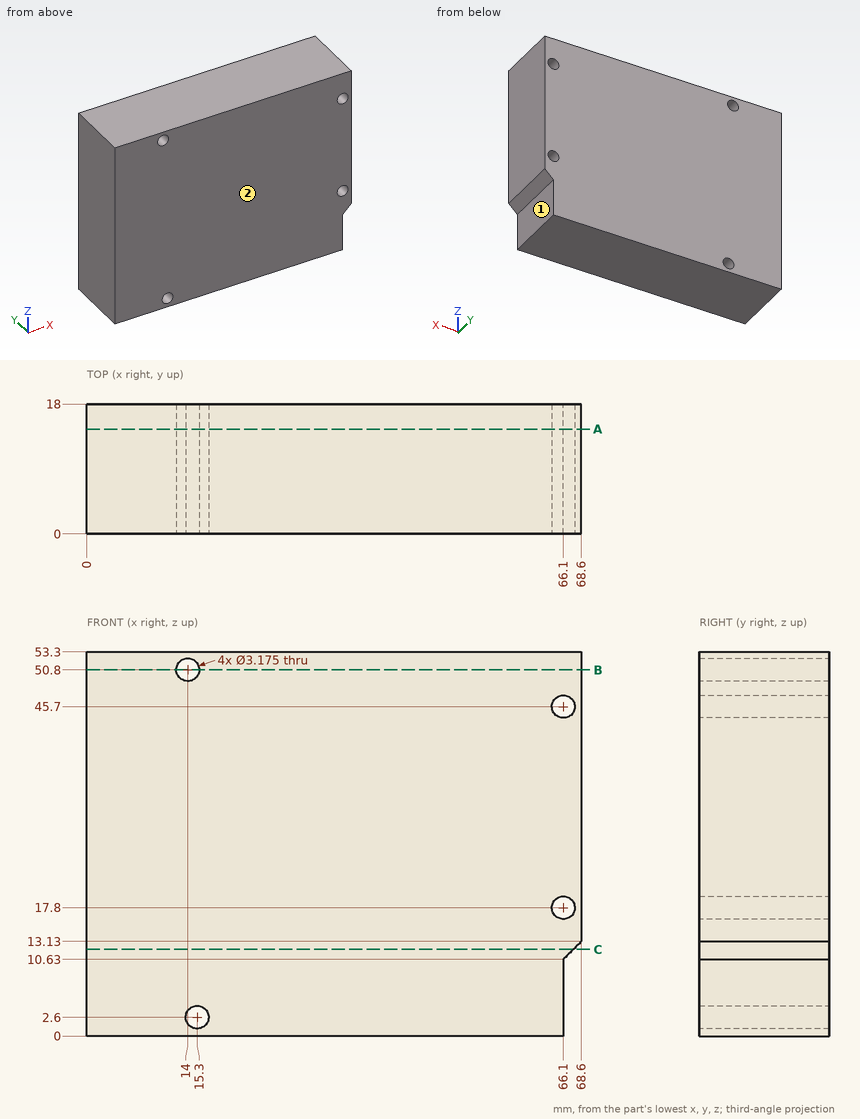
Geometry: see drawing. Coordinates: mm, zero at the bounding-box minimum. A direction names the side the tool comes from. Coordinates: 2 decimals unless noted, no trailing zeros. Write each loop counter-clockwise with the first axis right and the second up, starting at its lowest first coordinate (ties: lowest second). Pieces come first, ordered by that corner, then holes.
1) Set-up query: the marked faces 1 and 2. Return all of +Z, -Z, +X, -X, +Y, -Y with unobstructed straight access to the full face (end or side cutting, diameter ignored); none if empty.
2) Material intervals for line 1 along X through (y, z) = (6.25, 50.8); line 2 along X through (y, z) = (5.75, 2.6); line 3 along Z through (x, y) = (65, 15) (1 decimal), sorted ascending.
3) Section B-B on z = 50.8. Output: boundary loops of the cut face in (x, y).
4) Section C-C on z = 12. Output: boundary loops of the cut face in (x, y).
5) Section A-A on y = 14.5. Output: boundary loops of the cut face in (x, z) (1 decimal).
6) Pin query (flat end, axial travel): pin 1 Ø2.5 at (x, z) = (15.3, 2.6) entering from -Y. Return the tip coordinate at first contact, or that it passes through.
Check result:
1. face 1: -Z, +X, +Y, -Y
1. face 2: +Z, -Z, +X, -X, -Y
2. line 1: x = 0 to 12.41, 15.59 to 68.6
2. line 2: x = 0 to 13.71, 16.89 to 66.1
2. line 3: z = 0 to 16.7, 18.9 to 44.6, 46.8 to 53.3
3. outline: (0, 0) - (12.41, 0) - (12.41, 18) - (0, 18) - close; (15.59, 0) - (68.6, 0) - (68.6, 18) - (15.59, 18) - close
4. outline: (0, 0) - (67.47, 0) - (67.47, 18) - (0, 18) - close
5. outline: (0, 0) - (66.1, 0) - (66.1, 10.6) - (68.6, 13.1) - (68.6, 53.3) - (0, 53.3) - close; hole circle Ø3.2 at (14, 50.8); hole circle Ø3.2 at (15.3, 2.6); hole circle Ø3.2 at (66.1, 17.8); hole circle Ø3.2 at (66.1, 45.7)
6. pin 1: passes through
